from build123d import *

# Parameters (mm, degrees)
RESSALTO_EXTRUS_O1_DEPTH = 130
ESBO_O2_R                = 3.35
RESSALTO_EXTRUS_O2_DEPTH = 1
ESBO_O3_R                = 3.1
RESSALTO_EXTRUS_O3_DEPTH = 5.4
FILETE1_R                = 0.5
RESSALTO_EXTRUS_O4_START = 1
ESBO_O4_R                = 3.35
RESSALTO_EXTRUS_O4_DEPTH = 1


with BuildPart() as part:
    # Esboço1 → Ressalto-extrusão1 (new body)
    with BuildSketch(Plane(origin=(0, 0, 0), x_dir=(1, 0, 0), z_dir=(0, 1, 0))):
        with BuildLine():
            Line((0.3, -3.695041723), (3.05, -2.107328483))
            ThreePointArc((3.05, -2.107328483), (3.269615242, -1.88771324), (3.35, -1.58771324))
            Line((3.35, -1.58771324), (3.35, 1.58771324))
            ThreePointArc((3.35, 1.58771324), (3.269615242, 1.88771324), (3.05, 2.107328483))
            Line((3.05, 2.107328483), (0.3, 3.695041723))
            ThreePointArc((0.3, 3.695041723), (0, 3.775426481), (-0.3, 3.695041723))
            Line((-0.3, 3.695041723), (-3.05, 2.107328483))
            ThreePointArc((-3.05, 2.107328483), (-3.269615242, 1.88771324), (-3.35, 1.58771324))
            Line((-3.35, 1.58771324), (-3.35, -1.58771324))
            ThreePointArc((-3.35, -1.58771324), (-3.269615242, -1.88771324), (-3.05, -2.107328483))
            Line((-3.05, -2.107328483), (-0.3, -3.695041723))
            ThreePointArc((-0.3, -3.695041723), (0, -3.775426481), (0.3, -3.695041723))
        make_face()
    extrude(amount=RESSALTO_EXTRUS_O1_DEPTH)

    # Esboço2 → Ressalto-extrusão2 (add)
    with BuildSketch(Plane(origin=(0, 130, 0), x_dir=(1, 0, 0), z_dir=(0, 1, 0))):
        with Locations(Location((0, 0, 0), (0, 0, 60))):
            Circle(ESBO_O2_R)
    extrude(amount=RESSALTO_EXTRUS_O2_DEPTH)

    # Esboço3 → Ressalto-extrusão3 (add)
    with BuildSketch(Plane(origin=(0, 131, 0), x_dir=(1, 0, 0), z_dir=(0, 1, 0))):
        with Locations(Location((0, 0, 0), (0, 0, 90))):
            Circle(ESBO_O3_R)
    extrude(amount=RESSALTO_EXTRUS_O3_DEPTH)

    # Filete1
    filete1_edges = [part.edges().sort_by_distance(p)[0] for p in [
        (0, 136.4, 3.1),
    ]]
    fillet(filete1_edges, radius=FILETE1_R)

    # Esboço4 → Ressalto-extrusão4 (add)
    with BuildSketch(Plane.XZ.offset(RESSALTO_EXTRUS_O4_START)):
        with Locations(Location((0, 0, 0), (0, 0, 300))):
            Circle(ESBO_O4_R)
    extrude(amount=-RESSALTO_EXTRUS_O4_DEPTH)

    # Esboço5 → Revolução1 (revolve)
    with BuildSketch(Plane.XY, mode=Mode.PRIVATE) as revolu_o1_sk:
        with BuildLine():
            Line((3.05, -1), (3.05, -3.5))
            ThreePointArc((3.05, -3.5), (2.884182518, -7.015607207), (2.388202336, -10.5))
            ThreePointArc((2.388202336, -10.5), (1.838385418, -13.484350504), (1.5, -16.5))
            Line((1.5, -16.5), (1.2, -16.5))
            ThreePointArc((1.2, -16.5), (0.8415304, -17.4728826), (0.7, -18.5))
            Line((0.7, -18.5), (0.7, -19.1))
            Line((0.7, -19.1), (0.3, -19.1))
            Line((0.3, -19.1), (0.3, -20.5))
            Line((0.3, -20.5), (0, -20.5))
            Line((0, -20.5), (0, -1))
            Line((0, -1), (3.05, -1))
        make_face()
    revolve(revolu_o1_sk.sketch.rotate(Axis((0, -1, 0), (0, -1, 0)), 180), axis=Axis((0, -1, 0), (0, -1, 0)))


solid = part.part
CAD build for the part. Positions are in the model's coordinates, mm. A direction names the side the tool comes from. Coordinates: 2 decimals unless noted, no trailing zeros. Loops run counter-clockwise (first coordinate to the right, second up) from the corner with the lowest first, then second, coordinate; pieces in that order, holes last. Notation, with made-up numbers: (-36, 48) -> (14, 48) arc R13 ccw to (14, 55) -> close; hole circle Ø2 at (80.5, 57.25). An arc over 180 degrees is marked (long way). One line per item, written item: value.
1. Slice it at A-A on y = 14.5. Write the cut outline in (x, z).
Answers:
outline: (-3.35, -1.59) arc R0.6 ccw to (-3.05, -2.11) -> (-0.3, -3.7) arc R0.6 ccw to (0.3, -3.7) -> (3.05, -2.11) arc R0.6 ccw to (3.35, -1.59) -> (3.35, 1.59) arc R0.6 ccw to (3.05, 2.11) -> (0.3, 3.7) arc R0.6 ccw to (-0.3, 3.7) -> (-3.05, 2.11) arc R0.6 ccw to (-3.35, 1.59) -> close
2. Which spindle directions (+Z, -Z, +X, -X, +Y, -Y) get a long thin tool onto all of the face, cutting with end or side? Do faces 1 (the face through (3.35, 64, 0)), 2 (the face through (0.73, -0.51, 3.27)), 3 (the face through (-0.931, 133.416, -2.957)). Say none if no direction does.
Answers:
face 1: +Z, -Z, +X, +Y, -Y
face 2: -Y
face 3: +Y
3. Flat gauge pins, fed straight in: P1, Ø0.9, axis at x = -0.5, z = 0, coming from the -Y side; P2, Ø2, axis at x = 1.5, y = 83, coming from the -Z side; P3, Ø0.5, axis at x = -2.5, z = -1.5, coming from the +Y side; P4, Ø1.5, axis at x = -2.5, y = 86, coming from the +Z side. Where does each tip first touch, or does it go through?
Answers:
P1: stops at y = -20.5
P2: stops at z = -3.58
P3: stops at y = 136.4
P4: stops at z = 2.86
4. Drill centre lines: line 1 (Y direction, x = -0.25, z = 0.25); line 2 (X direction, y = 30, z = 1.75); line 3 (Z direction, x = 3, y = 91). Where is each one in solid material? Low to high. Write a range as [from, to].
Answers:
line 1: y = [-19.1, 136.4]
line 2: x = [-3.33, 3.33]
line 3: z = [-2.14, 2.14]
